```python
from build123d import *

# Parameters (mm, degrees)
SKETCH1_W           = 185
SKETCH1_H           = 40
BOSS_EXTRUDE1_DEPTH = 20
SKETCH2_W           = 8.25003803
SKETCH2_H           = 32.854024614
CUT_EXTRUDE1_DEPTH  = 188.149672722
FILLET1_R           = 5


with BuildPart() as part:
    # Sketch1 → Boss-Extrude1 (new body)
    with BuildSketch(Plane.XY):
        Rectangle(SKETCH1_W, SKETCH1_H)
    extrude(amount=BOSS_EXTRUDE1_DEPTH)

    # Sketch2 → Cut-Extrude1 (cut, through all)
    with BuildSketch(Plane(origin=(92.5, 0, 0), x_dir=(0, 0, -1), z_dir=(1, 0, 0))):
        with Locations((-20, 0)):
            Rectangle(SKETCH2_W, SKETCH2_H)
        Rectangle(SKETCH2_W, SKETCH2_H)
    extrude(amount=-CUT_EXTRUDE1_DEPTH, mode=Mode.SUBTRACT)

    # Fillet1
    # the kernel refuses this fillet: 5 mm, written as the material it adds along each edge
    with BuildSketch(Plane(origin=(92.5, 16.427012307, 4.125019015), x_dir=(0, 0, -1), z_dir=(-1, 0, 0)), Plane(origin=(92.5, -16.427012307, 15.874980985), x_dir=(0, 0, 1), z_dir=(-1, 0, 0))) as fillet1_piece_1:
        with BuildLine():
            CenterArc((5, 4.922845547), FILLET1_R, 180, 79.921563206)
            Line((0, 4.922845547), (-0.1, 4.922845547))
            Line((-0.1, 4.922845547), (-0.1, 0))
            Line((-0.1, 0), (0, -0.1))
            ThreePointArc((0, -0.1), (2.062509508, -0.1), (4.107519396, -0.098456911))
            Line((4.107519396, -0.098456911), (4.125019015, 0))
        make_face()
    extrude(amount=185)
    with BuildSketch(Plane(origin=(92.5, -16.427012307, 4.125019015), x_dir=(0, 1, 0), z_dir=(-1, 0, 0)), Plane(origin=(92.5, 16.427012307, 15.874980985), x_dir=(0, -1, 0), z_dir=(-1, 0, 0))) as fillet1_piece_2:
        with BuildLine():
            CenterArc((4.922845547, 5), FILLET1_R, 190.078436794, 79.921563206)
            Line((0, 4.125019015), (-0.098456911, 4.107519396))
            ThreePointArc((-0.098456911, 4.107519396), (-0.1, 2.062509508), (-0.1, 0))
            Line((-0.1, 0), (0, -0.1))
            Line((0, -0.1), (4.922845547, -0.1))
            Line((4.922845547, -0.1), (4.922845547, 0))
        make_face()
    extrude(amount=185)


solid = part.part
```
Input: part model. Units: mm. Frame: model coordinates. A direction names the side the tool comes from. Coordinates: 2 decimals unless noted, no trailing zeros. Loops run counter-clockwise (first coordinate to the right, second up) from the corner with the lowest first, then second, coordinate; pieces in that order, holes last. Notation, with made-up numbers: M 43.25,87.5 L 52.25,87.5 A18 ccw 52.25,115.5 Z; hole C 70,63 d6. An arc over 180 degrees is marked long. Use a Markdown table: item, result. Add a question column.
1) Section C-C, the plane y = -3.5. Return the cut outline in (x, z).
2) Set-up query: faces 1 (the cylindrical face through (1.3, 14.75, 17.07)), 2 (the cylindrical face through (1.295, 14.678, 2.989)), 3 (the flat face through (-92.5, 0, 10)). Return all of +Z, -Z, +X, -X, +Y, -Y with unobstructed straight access to the full face (end or side cutting, diameter ignored); none if empty.
3) Draft query along Y for faces 4 (the flat face through (92.5, 0, 10)), 5 (the flat face through (-1, 20, 10)), 6 (the flat face through (-1, -20, 10)), 7 (the flat face through (1, 0, 15.875)). Return one class per face: +Y half, -Y half, draft (parallel to the pull), parting line (faces both ways), or undercut.
4) Section A-A, the plane x = -45.5. Return the cut outline in (y, z), plus the area to 3 significant figures.
5) Line query: L1, parallel to Z at x = -53.5, y = -8.5; L2, parallel to Y at x = 73, z = 17.75; L3, parallel to Y at x = 27, z = 17. Output: solid intervals per line, ascending. Write a range as from..to.
6) Section B-B, the plane z = 18. Return the cut outline in (x, y), plus the area to 3 significant figures.
7) Pin query (flat end, axial travel): P1, Ø8, axis at y = 9, z = 17, coming from the +X side; P2, Ø10, axis at x = -22, y = 0.5, coming from the +Z side (3 decimals). Return the tip coordinate at first contact, or that it passes through.
Answer below:
| question | item | result |
|---|---|---|
| 1 | outline | M -92.5,4.13 L 92.5,4.13 L 92.5,15.87 L -92.5,15.87 Z |
| 2 | face 1 | +Z, +X, -X |
| 2 | face 2 | -Z, +X, -X |
| 2 | face 3 | +Z, -Z, -X, +Y, -Y |
| 3 | face 4 | draft |
| 3 | face 5 | +Y half |
| 3 | face 6 | -Y half |
| 3 | face 7 | undercut |
| 4 | outline | M -20,0 L -16.43,0 A5 cw -11.5,4.13 L 11.5,4.13 A5 cw 16.43,0 L 20,0 L 20,20 L 16.43,20 A5 cw 11.5,15.87 L -11.5,15.87 A5 cw -16.43,20 L -20,20 Z |
| 4 | area | 549 mm2 |
| 5 | L1 | 4.13..15.87 |
| 5 | L2 | -20..-15.41, 15.41..20 |
| 5 | L3 | -20..-14.66, 14.66..20 |
| 6 | outline | M -92.5,-20 L 92.5,-20 L 92.5,-15.59 L -92.5,-15.59 Z; M -92.5,15.59 L 92.5,15.59 L 92.5,20 L -92.5,20 Z |
| 6 | area | 1,630 mm2 |
| 7 | P1 | x = 92.5 |
| 7 | P2 | z = 15.875 |
